Geometry: final body of the model. Coordinates: model frame, mm. Face numbers are marked on the shaded views. A direction names the side the tool comes from. Give positions to 0.01 mm unless a question says otherwise; leave off trailing zeros. Loops run counter-clockwise (first coordinate to the right, second up) from the corner with the lowest first, then second, coordinate; pieces in that order, holes last. Notation, with made-up numbers: (77.25, -36.5) -> (131.25, -36.5) arc R21 ccw to (131.25, -26.5) -> close; hole circle Ø8 at (85, -7). An arc over 180 degrees is marked (long way). Answer in a Markdown table with one row per item. Add a question column.
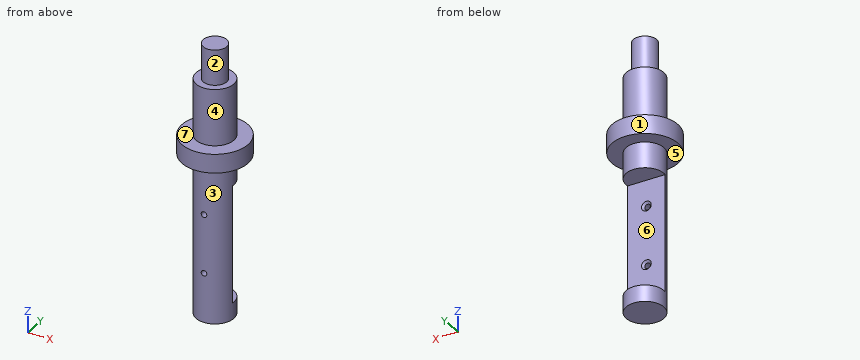
from build123d import *

# Parameters (mm, degrees)
SKETCH1_R                       = 8
BOSS_EXTRUDE1_DEPTH             = 34
SKETCH2_R                       = 14
BOSS_EXTRUDE2_DEPTH             = 8
SKETCH3_R                       = 8
BOSS_EXTRUDE3_DEPTH             = 24
SKETCH4_R                       = 5
BOSS_EXTRUDE4_DEPTH             = 15
SKETCH5_W                       = 50
SKETCH5_H                       = 13.172720446
CUT_EXTRUDE1_DEPTH              = 15
CUT_EXTRUDE1_DEPTH_BACK         = 15
F_4_48_TAPPED_HOLE1_D           = 2.3749
F_4_48_TAPPED_HOLE1_DEPTH       = 10.35
F_4_48_TAPPED_HOLE1_CSINK_D     = 4.1148
F_4_48_TAPPED_HOLE1_CSINK_ANGLE = 90
F_4_48_TAPPED_HOLE1_TIP         = 0.713491942


with BuildPart() as part:
    # Sketch1 → Boss-Extrude1 (new body, symmetric)
    with BuildSketch(Plane.XY):
        Circle(SKETCH1_R)
    extrude(amount=BOSS_EXTRUDE1_DEPTH, both=True)

    # Sketch2 → Boss-Extrude2 (add)
    with BuildSketch(Plane.XY.offset(34)):
        Circle(SKETCH2_R)
    extrude(amount=BOSS_EXTRUDE2_DEPTH)

    # Sketch3 → Boss-Extrude3 (add)
    with BuildSketch(Plane.XY.offset(42)):
        Circle(SKETCH3_R)
    extrude(amount=BOSS_EXTRUDE3_DEPTH)

    # Sketch4 → Boss-Extrude4 (add)
    with BuildSketch(Plane.XY.offset(66)):
        Circle(SKETCH4_R)
    extrude(amount=BOSS_EXTRUDE4_DEPTH)

    # Sketch5 → Cut-Extrude1 (cut, two sides)
    with BuildSketch(Plane(origin=(0, 0, 0), x_dir=(0, 0, -1), z_dir=(1, 0, 0))) as cut_extrude1_sk:
        with Locations((2, 5.586360223)):
            Rectangle(SKETCH5_W, SKETCH5_H)
    extrude(amount=CUT_EXTRUDE1_DEPTH, mode=Mode.SUBTRACT)
    extrude(cut_extrude1_sk.sketch, amount=-CUT_EXTRUDE1_DEPTH_BACK, mode=Mode.SUBTRACT)

    # #4-48 Tapped Hole1
    with Locations(Plane(origin=(0, -1, 0), x_dir=(1, 0, 0), z_dir=(0, 1, 0))):
        with Locations((0, -12), (0, 13)):
            CounterSinkHole(F_4_48_TAPPED_HOLE1_D / 2, F_4_48_TAPPED_HOLE1_CSINK_D / 2, depth=F_4_48_TAPPED_HOLE1_DEPTH, counter_sink_angle=F_4_48_TAPPED_HOLE1_CSINK_ANGLE)
            with Locations((0, 0, -(F_4_48_TAPPED_HOLE1_DEPTH + F_4_48_TAPPED_HOLE1_TIP / 2))):  # 118° drill point
                Cone(0, F_4_48_TAPPED_HOLE1_D / 2, F_4_48_TAPPED_HOLE1_TIP, mode=Mode.SUBTRACT)


solid = part.part
(1) Reachability of the marked faces 1, 2 and 3 from +Z, -Z, +X, -X, +Y, -Y: full face, straight path, thin tool, end or side. Return the list, or none.
(2) Material intervals for line 1 along Z through (x, y) = (0, -6.5); line 2 along Z through (x, y) = (0, -3.25); line 3 along X through (y, z) = (-6.25, -13), sorted ascending. Write a range as from..to.
(3) Cut plane D-D on z = -24. Return the cut outline in (x, y).
(4) Draft query along Z for the marked faces 4, 5, 6 and 7. Return one class per face: +Z half, -Z half, draft (parallel to the pull), parting line (faces both ways), or undercut.
(5) Cut plane C-C on x = 6.75. Return the cut outline in (y, z), then the cut area to 3 significant figures.
(6) Cut plane B-B on z = 12. Return the cut outline in (x, y), then the cut area to 3 significant figures.
(7) Pin query (flat end, axial travel): pin 1 Ø12 at (x, y) = (-7, 9) entering from +Z; pin 2 Ø2 at (y, z) = (9.5, 52) entering from -X; pin 3 Ø3 at (x, z) = (-6, 67) entering from +Y; pin 4 Ø4 at (x, z) = (0, -13) entering from -Y. Return the tip coordinate at first contact, or that it passes through.
(8) Cut plane A-A on y = 0. Return the cut outline in (x, z).
Answer list:
| question | item | result |
|---|---|---|
| 1 | face 1 | +Z, -Z |
| 1 | face 2 | +Z |
| 1 | face 3 | -Z |
| 2 | line 1 | z = -34..-14.19, -11.81..10.81, 13.19..66 |
| 2 | line 2 | z = -34..-14.19, -11.81..10.81, 13.19..81 |
| 2 | line 3 | x = -4.99..-1.19, 1.19..4.99 |
| 3 | outline | (-7.94, -1) arc R8 ccw to (7.94, -1) -> close |
| 4 | face 4 | draft |
| 4 | face 5 | -Z half |
| 4 | face 6 | undercut |
| 4 | face 7 | +Z half |
| 5 | outline | (-12.27, 34) -> (-4.29, 34) -> (-4.29, -34) -> (4.29, -34) -> (4.29, -27) -> (-1, -27) -> (-1, 23) -> (4.29, 23) -> (4.29, 34) -> (12.27, 34) -> (12.27, 42) -> (4.29, 42) -> (4.29, 66) -> (-4.29, 66) -> (-4.29, 42) -> (-12.27, 42) -> close |
| 5 | area | 722 mm² |
| 6 | outline | (-7.94, -1) arc R8 ccw to (-1.19, -7.91) -> (-1.19, -1.87) -> (-2.06, -1) -> close; (1.19, -7.91) arc R8 ccw to (7.94, -1) -> (2.06, -1) -> (1.19, -1.87) -> close |
| 6 | area | 67.3 mm² |
| 7 | pin 1 | stops at z = 66 |
| 7 | pin 2 | passes through |
| 7 | pin 3 | stops at y = 6.34 |
| 7 | pin 4 | stops at y = -8 |
| 8 | outline | (-14, 34) -> (-8, 34) -> (-8, 23) -> (8, 23) -> (8, 34) -> (14, 34) -> (14, 42) -> (8, 42) -> (8, 66) -> (5, 66) -> (5, 81) -> (-5, 81) -> (-5, 66) -> (-8, 66) -> (-8, 42) -> (-14, 42) -> close; (-8, -34) -> (8, -34) -> (8, -27) -> (-8, -27) -> close |
